```python
from build123d import *
from OCP.BRepFilletAPI import BRepFilletAPI_MakeChamfer

# Parameters (mm, degrees)
SKETCH_1_W       = 24.2
SKETCH_1_H       = 20.2
EXTRUDE_1_DEPTH  = 11.5
EXTRUDE_2_DEPTH  = 2
FILLET_1_R       = 2
EXTRUDE_3_DEPTH  = 0.1
CHAMFER_1_SIZE   = 4
CHAMFER_1_SIZE_2 = 1.07179677
CHAMFER_3_SIZE   = 1
CHAMFER_3_SIZE2  = 2.43937374
FILLET_2_R       = 2


with BuildPart() as part:
    # 草图1 → 凸台-拉伸1 (new body)
    with BuildSketch(Plane(origin=(0, 0, 0), x_dir=(1, 0, 0), z_dir=(0, 1, 0))):
        with Locations((12.1, 10.1)):
            Rectangle(SKETCH_1_W, SKETCH_1_H)
    extrude(amount=EXTRUDE_1_DEPTH)

    # 草图2 → 凸台-拉伸2 (add)
    # profile 1 of 2: a face of its own
    with BuildSketch(Plane.XZ):
        with BuildLine():
            Line((17.1, 0), (7.1, 0))
            Line((7.1, 0), (7.1, 3))
            ThreePointArc((7.1, 3), (7.978679656, 5.121320344), (10.1, 6))
            Line((10.1, 6), (14.1, 6))
            ThreePointArc((14.1, 6), (16.221320344, 5.121320344), (17.1, 3))
            Line((17.1, 3), (17.1, 0))
        make_face()
        with BuildLine():
            Line((14.1, 1.5), (10.1, 1.5))
            ThreePointArc((10.1, 1.5), (8.6, 3), (10.1, 4.5))
            Line((10.1, 4.5), (14.1, 4.5))
            ThreePointArc((14.1, 4.5), (15.6, 3), (14.1, 1.5))
        make_face(mode=Mode.SUBTRACT)
    # profile 2 of 2: a face of its own
    with BuildSketch(Plane.XZ):
        with BuildLine():
            Line((7.1, -23.2), (7.1, -20.2))
            Line((7.1, -20.2), (17.1, -20.2))
            Line((17.1, -20.2), (17.1, -23.2))
            ThreePointArc((17.1, -23.2), (16.221320344, -25.321320344), (14.1, -26.2))
            Line((14.1, -26.2), (10.1, -26.2))
            ThreePointArc((10.1, -26.2), (7.978679656, -25.321320344), (7.1, -23.2))
        make_face()
        with BuildLine():
            Line((14.1, -21.7), (10.1, -21.7))
            ThreePointArc((10.1, -21.7), (8.6, -23.2), (10.1, -24.7))
            Line((10.1, -24.7), (14.1, -24.7))
            ThreePointArc((14.1, -24.7), (15.6, -23.2), (14.1, -21.7))
        make_face(mode=Mode.SUBTRACT)
    extrude(amount=-EXTRUDE_2_DEPTH)

    # 圆角1
    fillet_1_edges = [part.edges().sort_by_distance(p)[0] for p in [
        (7.1, 1, -20.2),
        (17.1, 1, -20.2),
        (17.1, 1, 0),
        (7.1, 1, 0),
    ]]
    fillet(fillet_1_edges, radius=FILLET_1_R)

    # 草图3 → 凸台-拉伸3 (add)
    with BuildSketch(Plane(origin=(0, 11.5, 0), x_dir=(1, 0, 0), z_dir=(0, 1, 0))):
        with BuildLine():
            Line((5.1, 13.6), (19.1, 13.6))
            ThreePointArc((19.1, 13.6), (22.6, 10.1), (19.1, 6.6))
            Line((19.1, 6.6), (5.1, 6.6))
            ThreePointArc((5.1, 6.6), (1.6, 10.1), (5.1, 13.6))
        make_face()
    extrude(amount=EXTRUDE_3_DEPTH)

    # 倒角1
    # the kernel refuses this chamfer: 4, 1.07179677 mm, written as the material it takes off along each edge
    with BuildSketch(Plane(origin=(24.2, 11.5, 10.386886281), x_dir=(-1, 0, 0), z_dir=(0, 0, -1))) as chamfer_1_piece_1_section:
        Polygon((CHAMFER_1_SIZE, 0), (0, -CHAMFER_1_SIZE_2), (0, 0), align=None)
    chamfer_1_piece_1 = extrude(amount=40.973772562, mode=Mode.PRIVATE)
    chamfer_1_piece_1 = chamfer_1_piece_1 - Plane(origin=(19.1, 11.5, -10.1), x_dir=(0, 0, -1), z_dir=(0, -1, 0)) * Cylinder(3.5, 98, mode=Mode.PRIVATE)
    add(chamfer_1_piece_1, mode=Mode.SUBTRACT)
    with BuildSketch(Plane(origin=(34.586886281, 11.5, -20.2), x_dir=(0, 0, 1), z_dir=(-1, 0, 0))) as chamfer_1_piece_2:
        Polygon((CHAMFER_1_SIZE, 0), (0, -CHAMFER_1_SIZE_2), (0, 0), align=None)
    extrude(amount=44.973772562, mode=Mode.SUBTRACT)
    with BuildSketch(Plane(origin=(0, 11.5, -30.586886281), x_dir=(0, -1, 0), z_dir=(0, 0, 1))) as chamfer_1_piece_3_section:
        Polygon((CHAMFER_1_SIZE_2, 0), (0, CHAMFER_1_SIZE), (0, 0), align=None)
    chamfer_1_piece_3 = extrude(amount=40.973772562, mode=Mode.PRIVATE)
    chamfer_1_piece_3 = chamfer_1_piece_3 - Plane(origin=(5.1, 11.5, -10.1), x_dir=(0, 0, 1), z_dir=(0, -1, 0)) * Cylinder(3.5, 98, mode=Mode.PRIVATE)
    add(chamfer_1_piece_3, mode=Mode.SUBTRACT)
    with BuildSketch(Plane(origin=(-10.386886281, 11.5, 0), x_dir=(0, -1, 0), z_dir=(1, 0, 0))) as chamfer_1_piece_4:
        Polygon((CHAMFER_1_SIZE_2, 0), (0, CHAMFER_1_SIZE), (0, 0), align=None)
    extrude(amount=44.973772562, mode=Mode.SUBTRACT)

    # 倒角3: one chamfer whose edges measure the first distance from different faces: ONE call of the kernel's chamfer builder (chamfer() names one face for all edges)
    chamfer_3_edges_1 = [part.edges().sort_by_distance(p)[0] for p in [
        (22.2, 10.964101615, -2),
        (22.2, 10.964101615, -18.2),
    ]]
    chamfer_3_side_1 = [part.faces().sort_by_distance(p)[0] for p in [
        (22.621463638, 10.851170773, -10.1),
    ]]
    chamfer_3_edges_2 = [part.edges().sort_by_distance(p)[0] for p in [
        (2, 10.964101615, -2),
        (2, 10.964101615, -18.2),
    ]]
    chamfer_3_side_2 = [part.faces().sort_by_distance(p)[0] for p in [
        (1.578536362, 10.851170773, -10.1),
    ]]
    chamfer_3 = BRepFilletAPI_MakeChamfer(part.part.solid().wrapped)
    for e in chamfer_3_edges_1:
        chamfer_3.Add(CHAMFER_3_SIZE, CHAMFER_3_SIZE2, e.wrapped, chamfer_3_side_1[0].wrapped)  # the first distance lies on this face
    for e in chamfer_3_edges_2:
        chamfer_3.Add(CHAMFER_3_SIZE, CHAMFER_3_SIZE2, e.wrapped, chamfer_3_side_2[0].wrapped)  # the first distance lies on this face
    add(Compound.cast(chamfer_3.Shape()), mode=Mode.REPLACE)

    # 圆角2
    fillet_2_edges = [part.edges().sort_by_distance(p)[0] for p in [
        (0, 5.081990675, 0),
        (0, 5.081990675, -20.2),
        (24.2, 5.081990675, -20.2),
        (24.2, 5.081990675, 0),
    ]]
    fillet(fillet_2_edges, radius=FILLET_2_R)


solid = part.part
```
Here's how the part is built. I have some questions about the finished solid (model axes, mm). A direction names the side the tool comes from. Coordinates: 2 decimals unless noted, no trailing zeros. Loops run counter-clockwise (first coordinate to the right, second up) from the corner with the lowest first, then second, coordinate; pieces in that order, holes last. Notation, with made-up numbers: (62.25, -10.75) - (111.25, -10.75) arc R22 ccw to (111.25, 21.25) - close; hole circle Ø8 at (-3, 54). An arc over 180 degrees is marked (long way). Answer as CSV lines item,"result".
Q1. If I drill on L1, parallel to Y at x = 10, z = -6.5; L2, parallel to Y at x = 8.25, z = -22; L3, parallel to Z at x = 13.75, y = 10, over which ranges is the centre line in solid material (lowest first)? Write a range as [from, to].
Response:
L1,"[0, 11.5]"
L2,"[0, 2]"
L3,"[-20.2, 0]"
Q2. If we section it at D-D, the plane x = 9.75: Write out the boundary of the cut face in (y, z).
Response:
outline,"(0, -26.18) - (2, -26.18) - (2, -24.66) - (0, -24.66) - close; (0, -21.74) - (2, -21.74) - (2, -20.2) - (10.43, -20.2) - (11.5, -16.2) - (11.5, -13.6) - (11.6, -13.6) - (11.6, -6.6) - (11.5, -6.6) - (11.5, -4) - (10.43, 0) - (2, 0) - (2, 1.54) - (0, 1.54) - close; (0, 4.46) - (2, 4.46) - (2, 5.98) - (0, 5.98) - close"
Q3. For pin 1 (3 mm diameter, centred on x = 10, z = -15.5, fed in from +Y); pin 2 (3 mm diameter, centred on x = 9.5, z = -22, fed in from +Y); pin 3 (5 mm diameter, centred on x = 12, z = 2, fed in from +Y), each with a flat end and sliding along its axis, tell me the tip position at first contact or that it passes through.
Response:
pin 1,"y = 11.5"
pin 2,"y = 2"
pin 3,"y = 10.56"
Q4. If we section it at B-B, the plane y = 4.25: Write out the boundary of the cut face in (x, z).
Response:
outline,"(0, -18.2) arc R2 ccw to (2, -20.2) - (22.2, -20.2) arc R2 ccw to (24.2, -18.2) - (24.2, -2) arc R2 ccw to (22.2, 0) - (2, 0) arc R2 ccw to (0, -2) - close"
Q5. For faces 1 (the face through (12, 1, 4.5)), 2 (the face through (1.6, 11.4, -10)), 3 (the face through (17.1, 1, 2.5)), 4 (the face through (17.1, 1, -23)), which set-ups out of +Z, -Z, +X, -X, +Y, -Y let a thin tool reach every point of the face, with its end or its side?
Response:
face 1,"+Y, -Y"
face 2,"-X, +Y"
face 3,"+Z, +X, +Y, -Y"
face 4,"-Z, +X, +Y, -Y"
Q6. If we section it at C-C, the plane z = -14: Write out the boundary of the cut face in (x, y).
Response:
outline,"(0, 0) - (24.2, 0) - (24.2, 10.43) - (20.2, 11.5) - (4, 11.5) - (0, 10.43) - close"
Q7. If we section it at A-A, the plane x = 12.5: Write out the boundary of the cut face in (y, z), and give its area (3 significant figures).
Response:
outline,"(0, -26.2) - (2, -26.2) - (2, -24.7) - (0, -24.7) - close; (0, -21.7) - (2, -21.7) - (2, -20.2) - (10.43, -20.2) - (11.5, -16.2) - (11.5, -13.6) - (11.6, -13.6) - (11.6, -6.6) - (11.5, -6.6) - (11.5, -4) - (10.43, 0) - (2, 0) - (2, 1.5) - (0, 1.5) - close; (0, 4.5) - (2, 4.5) - (2, 6) - (0, 6) - close"
area,"241 mm2"
Q8. We'd pull the mould along Z, two halves only. Please class faces 5 (the face through (12, 1, -26.2)), 6 (the face through (8.6, 1, -23.2)), 7 (the face through (12, 11.6, -10)): pulls with the +Z half, pulls with the -Z half, needs draft (parallel to the pull), parting line crosses it, or undercut.
Response:
face 5,"pulls with the -Z half"
face 6,"undercut"
face 7,"needs draft"
